Answer from the drawing. Dimensions are ordinates in mm from the lowest x, y and z of the part. A direction names the side the tool comes from. Give positions to 0.01 mm unless a question says otherwise; leave off trailing zeros. Loops run counter-clockwise (first coordinate to the right, second up) from the corner with the lowest first, then second, coordinate; pieces in that order, holes last.
(1) Find section B-B, the plane x = 55. Write down the section's boundary in (y, z).
(2) Determine the mould class of the marked faces 3, 4, 5 and 6 for opening direction X: pulls with the +X half, pulls with the -X half, needs draft (parallel to the pull), parting line crosses it, or undercut.
(3) Each of these flat-tipped pins is pushed along its axis until it touches: P1, Ø17, axis at x = 41, y = 19, coming from the -Z side; P2, Ø3.5, axis at x = 5, y = 5, coming from the -Z side. Where does it stop, or does it pass through?
(4) Find section C-C, the plane y = 32. Write down the section's boundary in (x, z).
(5) Find section A-A, the plane z = 4.5. Write down the section's boundary in (x, y).
(6) Find section D-D, the plane y = 4. Write down the section's boundary in (x, z) (1 decimal), then the cut area to 3 significant figures.
(7) Which of the six approach directions +Z, -Z, +X, -X, +Y, -Y give full straight-line access (tool end or side, diameter ignored) to the marked faces 1 and 2?
(8) Straight lines are drawn through the part: probe 1 along Y at (x, z) = (30, 17.5); probe 2 along X at (y, z) = (54, 2.75). For each, find the intervals that lie inside material, in ascending order.
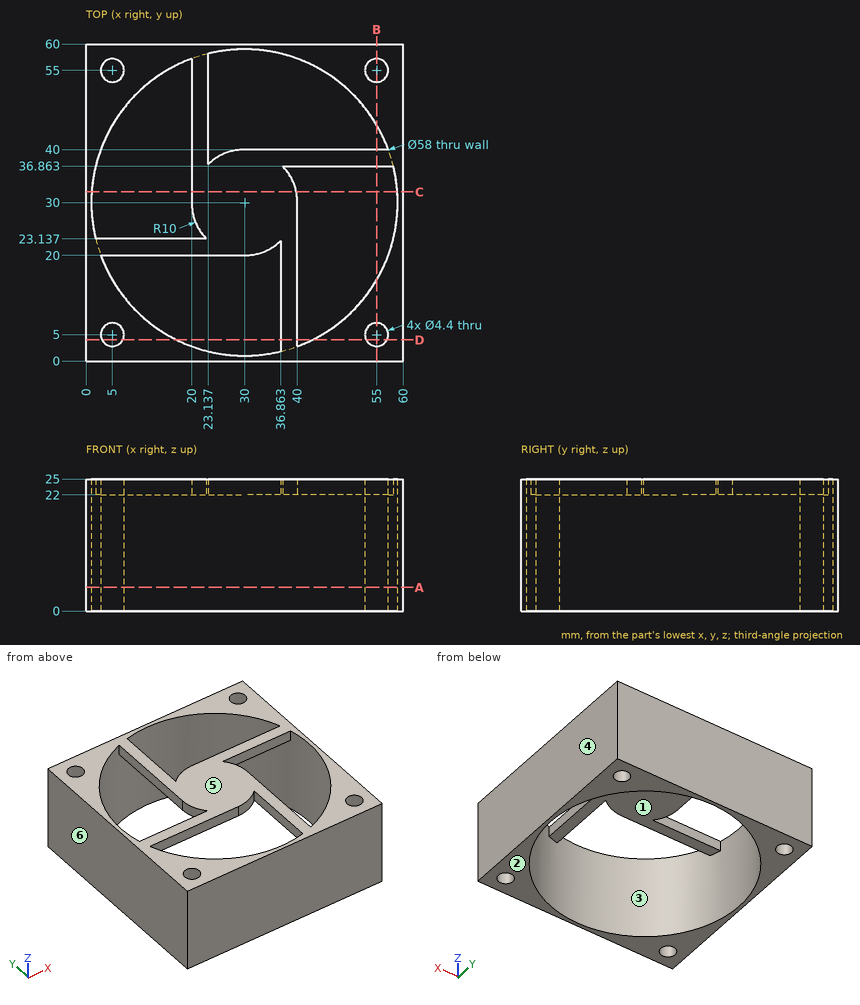
Entries:
1. outline: (0, 0) - (2.8, 0) - (2.8, 25) - (0, 25) - close; (7.2, 0) - (15.3, 0) - (15.3, 25) - (7.2, 25) - close; (36.86, 22) - (40, 22) - (40, 25) - (36.86, 25) - close; (44.7, 0) - (52.8, 0) - (52.8, 25) - (44.7, 25) - close; (57.2, 0) - (60, 0) - (60, 25) - (57.2, 25) - close
2. face 3: undercut
2. face 4: pulls with the +X half
2. face 5: needs draft
2. face 6: pulls with the -X half
3. P1: stops at z = 22
3. P2: passes through
4. outline: (0, 0) - (1.07, 0) - (1.07, 25) - (0, 25) - close; (20, 22) - (39.8, 22) - (39.8, 25) - (20, 25) - close; (58.93, 0) - (60, 0) - (60, 25) - (58.93, 25) - close
5. outline: (0, 0) - (60, 0) - (60, 60) - (0, 60) - close; hole circle Ø58 at (30, 30); hole circle Ø4.4 at (5, 5); hole circle Ø4.4 at (5, 55); hole circle Ø4.4 at (55, 5); hole circle Ø4.4 at (55, 55)
6. outline: (0, 0) - (3, 0) - (3, 25) - (0, 25) - close; (7, 0) - (17.2, 0) - (17.2, 25) - (7, 25) - close; (36.9, 22) - (40, 22) - (40, 25) - (36.9, 25) - close; (42.8, 0) - (53, 0) - (53, 25) - (42.8, 25) - close; (57, 0) - (60, 0) - (60, 25) - (57, 25) - close
6. area: 671 mm2
7. face 1: -Z
7. face 2: -Z, +X, -X, +Y, -Y
8. probe 1: y = 0 to 1, 59 to 60
8. probe 2: x = 0 to 3.04, 6.96 to 13.72, 46.28 to 53.04, 56.96 to 60
